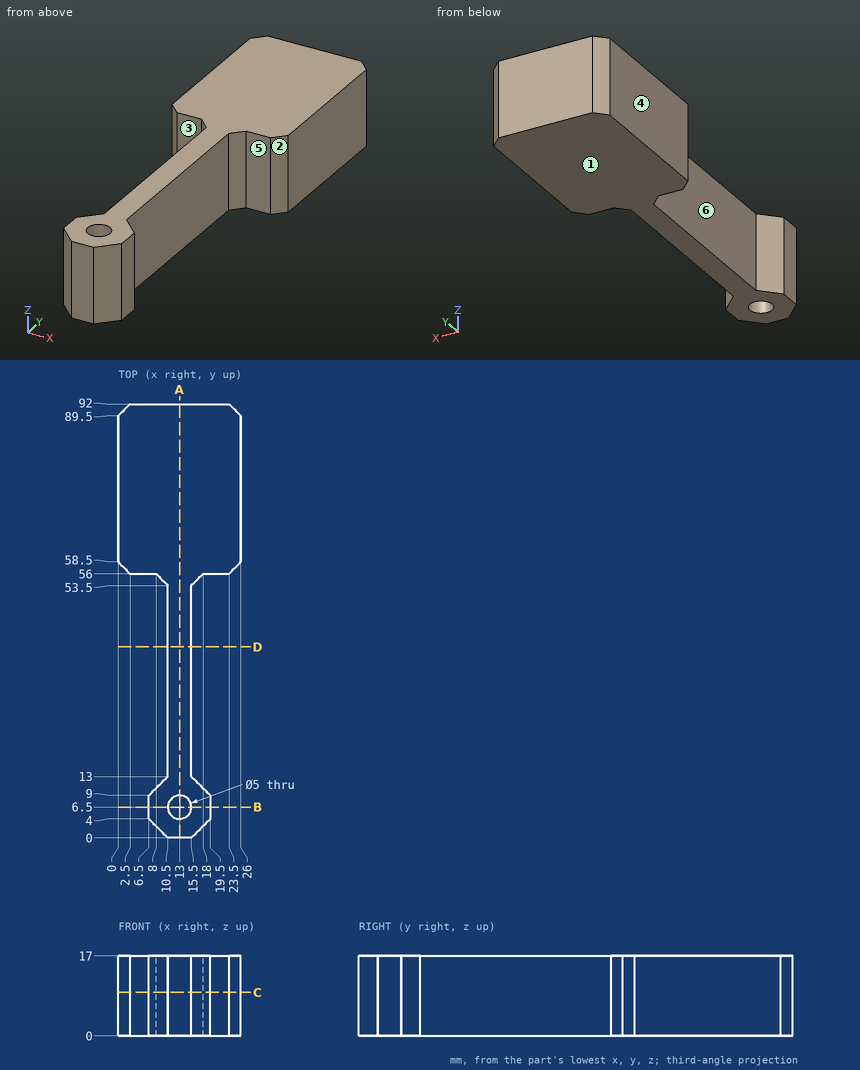
Can you work these out from the drawing? Everything is in mm from the part's minimum corner. A direction names the side the tool comes from. Give positions to 0.01 mm unless a question says otherwise; leave off trailing zeros. Loops run counter-clockwise (first coordinate to the right, second up) from the corner with the lowest first, then second, coordinate; pieces in that order, holes last. Notation, with made-up numbers: (21, 15.25) - (58, 15.25) arc R28 cw to (58, 37.25) - close; hole circle Ø2 at (-28.5, 51). An arc over 180 degrees is marked (long way). Answer as a JSON object with one key per item and string values.
Q1. Will these pins go through, and if not, where does the flat tip stop? P1, Ø4.5, axis at x = 5, z = 5.5, coming from the -Y side; P2, Ø1.5, axis at x = 16, y = 16, coming from the -Z side; P3, Ø5, axis at y = 40, z = 12, coming from the -X side; P4, Ø2.5, axis at y = 6.5, z = 12, coming from the -X side.
Geometry says:
{"P1": "y = 3.25", "P2": "z = 0", "P3": "x = 10.5", "P4": "x = 6.5"}
Q2. Imagine slicing it at D-D on y = 40.5. Write out the boundary of the cut face in (x, z).
Geometry says:
{"outline": "(10.5, 0) - (15.5, 0) - (15.5, 17) - (10.5, 17) - close"}
Q3. Which directions (+Z, -Z, +X, -X, +Y, -Y) give clear straight access to the entire face, cutting with the end or side of a thin tool? Please do the marked faces 4, 5 and 6.
Geometry says:
{"face 4": "+Z, -Z, -X, +Y, -Y", "face 5": "+Z, -Z, +X", "face 6": "+Z, -Z, -X"}
Q4. If I drill on L1, parallel to Y at x = 13, z = 11; L2, parallel to X at y = 19.5, z = 4.5; L3, parallel to Y at x = 8.5, z = 4, over which ranges is the centre line in solid material (lowest first)?
Geometry says:
{"L1": "0 to 4, 9 to 92", "L2": "10.5 to 15.5", "L3": "2 to 11, 55.5 to 92"}
Q5. Imagine slicing it at B-B on y = 6.5. Write out the boundary of the cut face in (x, z), plus the area to 3 significant figures.
Geometry says:
{"outline": "(6.5, 0) - (10.5, 0) - (10.5, 17) - (6.5, 17) - close; (15.5, 0) - (19.5, 0) - (19.5, 17) - (15.5, 17) - close", "area": "136 mm²"}
Q6. Imagine slicing it at A-A on x = 13. Write out the boundary of the cut face in (y, z), plus the area to 3 significant figures.
Geometry says:
{"outline": "(0, 0) - (4, 0) - (4, 17) - (0, 17) - close; (9, 0) - (92, 0) - (92, 17) - (9, 17) - close", "area": "1,480 mm²"}
Q7. If we mould it in two halves opening along Y, with no side actions, what happens to the marked faces 1, 2 and 3? For each: pulls with the +Y half, pulls with the -Y half, needs draft (parallel to the pull), parting line crosses it, or undercut.
Geometry says:
{"face 1": "needs draft", "face 2": "pulls with the -Y half", "face 3": "undercut"}
Q8. Imagine slicing it at C-C on z = 9.25. Write out the boundary of the cut face in (x, y), plus the area to 3 significant figures.
Geometry says:
{"outline": "(0, 58.5) - (2.5, 56) - (8, 56) - (10.5, 53.5) - (10.5, 13) - (6.5, 9) - (6.5, 4) - (10.5, 0) - (15.5, 0) - (19.5, 4) - (19.5, 9) - (15.5, 13) - (15.5, 53.5) - (18, 56) - (23.5, 56) - (26, 58.5) - (26, 89.5) - (23.5, 92) - (2.5, 92) - (0, 89.5) - close; hole circle Ø5 at (13, 6.5)", "area": "1,260 mm²"}
